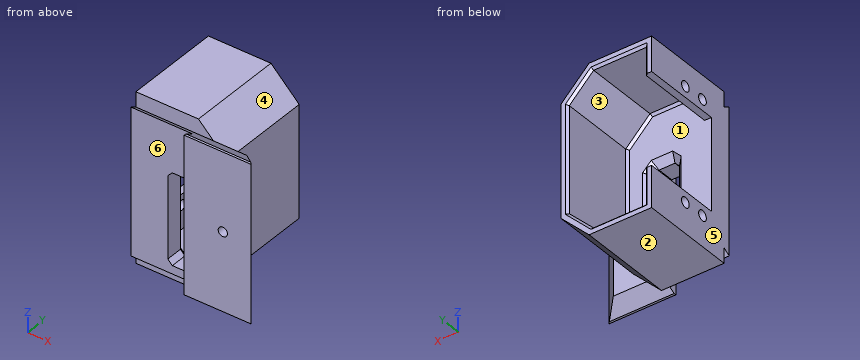
from build123d import *

# Parameters (mm, degrees)
MAIN_FACE_EXTRUDE_DEPTH              = 7.4
MAIN_WALLS_EXTRUDE_DEPTH             = 35
MAIN_WALLS_LOWER_CHAMFER_SIZE        = 1
MAIN_WALLS_ENTRY_CHAMFER_SIZE        = 1
SKETCH4_W                            = 3
SKETCH4_H                            = 40.5
SERVO_MOUNT_CUT_DEPTH                = 35
SERVO_MOUNT_HOLES_REACH              = 72.134
SKETCH5_R                            = 2.25
MOUNT_DOVETAIL_DEPTH                 = 56.8
MOUNT_DOVETAIL_CHAMFER_SIZE          = 8
SKETCH9_W                            = 27.3
SKETCH9_H                            = 68.845299462
DOVETAIL_OFFSET_CUT_DEPTH            = 5
SKETCH10_R                           = 2.05
MOUNT_SCREW_HOLE_DEPTH               = 69.359344643
SKETCH11_R                           = 3.5
MOUNT_SCREW_COUNTERSINK_DEPTH        = 3
MOUNT_SCREW_COUNTERSINK_CHAMFER_SIZE = 1
GEAR_CUT_DEPTH                       = 65.033116432
GEAR_ENTRY_CHAMFER_SIZE              = 3


# Some blends are built 0.0001 mm under size
with BuildPart() as part:
    # Sketch1 → Main Face Extrude (new body)
    with BuildSketch(Plane(origin=(0, 0, 0), x_dir=(1, 0, 0), z_dir=(0, 1, 0))):
        Polygon((-20, 35), (7.542640687, 35), (20, 22.542640687), (20, -26.542640687), (7.542640687, -39), (-20, -39), align=None)
    extrude(amount=MAIN_FACE_EXTRUDE_DEPTH)

    # Sketch3 → Main Walls Extrude (add)
    with BuildSketch(Plane(origin=(0, 7.4, 0), x_dir=(1, 0, 0), z_dir=(0, 1, 0))):
        Polygon((-20, 35), (-20, -39), (7.542640687, -39), (20, -26.542640687), (20, 22.542640687), (7.542640687, 35), align=None)
        Polygon((-17, 32), (-17, -36), (6.3, -36), (17, -25.3), (17, 21.3), (6.3, 32), align=None, mode=Mode.SUBTRACT)
    extrude(amount=MAIN_WALLS_EXTRUDE_DEPTH)

    # Main Walls Lower Chamfer
    main_walls_lower_chamfer_edges = [part.edges().sort_by_distance(p)[0] for p in [
        (-5.35, 7.4, -32),
        (-5.35, 7.4, 36),
        (11.65, 7.4, 30.65),
        (17, 7.4, 2),
        (11.65, 7.4, -26.65),
    ]]
    chamfer(main_walls_lower_chamfer_edges, length=MAIN_WALLS_LOWER_CHAMFER_SIZE)

    # Main Walls Entry Chamfer
    main_walls_entry_chamfer_edges = [part.edges().sort_by_distance(p)[0] for p in [
        (-5.35, 42.4, -32),
        (-17, 42.4, 2),
        (-5.35, 42.4, 36),
        (11.65, 42.4, 30.65),
        (17, 42.4, 2),
        (11.65, 42.4, -26.65),
    ]]
    chamfer(main_walls_entry_chamfer_edges, length=MAIN_WALLS_ENTRY_CHAMFER_SIZE)

    # Sketch4 → Servo Mount Cut (cut)
    with BuildSketch(Plane(origin=(0, 42.4, 0), x_dir=(1, 0, 0), z_dir=(0, 1, 0))):
        with Locations((-18.5, -3.45)):
            Rectangle(SKETCH4_W, SKETCH4_H)
    extrude(amount=-SERVO_MOUNT_CUT_DEPTH, mode=Mode.SUBTRACT)

    # Sketch5 → Servo Mount Holes (cut, up to next)
    with BuildSketch(Plane.ZY.offset(20), mode=Mode.PRIVATE) as servo_mount_holes_sk1:
        with Locations((-21.6, 22.65)):
            Circle(SKETCH5_R)
    servo_mount_holes_tool1 = extrude(servo_mount_holes_sk1.sketch, amount=-SERVO_MOUNT_HOLES_REACH, mode=Mode.PRIVATE) & part.part
    # Sketch5 → Servo Mount Holes (cut, up to next)
    with BuildSketch(Plane.ZY.offset(20), mode=Mode.PRIVATE) as servo_mount_holes_sk2:
        with Locations((-21.6, 12.65)):
            Circle(SKETCH5_R)
    servo_mount_holes_tool2 = extrude(servo_mount_holes_sk2.sketch, amount=-SERVO_MOUNT_HOLES_REACH, mode=Mode.PRIVATE) & part.part
    # Sketch5 → Servo Mount Holes (cut, up to next)
    with BuildSketch(Plane.ZY.offset(20), mode=Mode.PRIVATE) as servo_mount_holes_sk3:
        with Locations((28.5, 22.65)):
            Circle(SKETCH5_R)
    servo_mount_holes_tool3 = extrude(servo_mount_holes_sk3.sketch, amount=-SERVO_MOUNT_HOLES_REACH, mode=Mode.PRIVATE) & part.part
    # Sketch5 → Servo Mount Holes (cut, up to next)
    with BuildSketch(Plane.ZY.offset(20), mode=Mode.PRIVATE) as servo_mount_holes_sk4:
        with Locations((28.5, 12.65)):
            Circle(SKETCH5_R)
    servo_mount_holes_tool4 = extrude(servo_mount_holes_sk4.sketch, amount=-SERVO_MOUNT_HOLES_REACH, mode=Mode.PRIVATE) & part.part
    add(servo_mount_holes_tool1.solids().sort_by_distance((-20, 22.65, -21.6))[0], mode=Mode.SUBTRACT)
    add(servo_mount_holes_tool2.solids().sort_by_distance((-20, 12.65, -21.6))[0], mode=Mode.SUBTRACT)
    add(servo_mount_holes_tool3.solids().sort_by_distance((-20, 22.65, 28.5))[0], mode=Mode.SUBTRACT)
    add(servo_mount_holes_tool4.solids().sort_by_distance((-20, 12.65, 28.5))[0], mode=Mode.SUBTRACT)

    # Sketch8 → Mount Dovetail (add)
    with BuildSketch(Plane.ZY.offset(20)):
        Polygon((-28.381197846, 0), (-32.422649731, -7), (-32.422649731, -8), (36.422649731, -8), (36.422649731, -7), (32.381197846, 0), align=None)
    extrude(amount=-MOUNT_DOVETAIL_DEPTH)

    # Mount Dovetail Chamfer
    mount_dovetail_chamfer_edges = [part.edges().sort_by_distance(p)[0] for p in [
        (36.8, 0, 2),
    ]]
    chamfer(mount_dovetail_chamfer_edges, length=MOUNT_DOVETAIL_CHAMFER_SIZE - 0.0001)  # a hair under: the kernel refuses the full size

    # Sketch9 → Dovetail Offset Cut (cut)
    with BuildSketch(Plane.XZ.offset(8)):
        with Locations((-6.35, 2)):
            Rectangle(SKETCH9_W, SKETCH9_H)
    extrude(amount=-DOVETAIL_OFFSET_CUT_DEPTH, mode=Mode.SUBTRACT)

    # Sketch10 → Mount Screw Hole (cut, through all)
    with BuildSketch(Plane(origin=(0, 0, 0), x_dir=(1, 0, 0), z_dir=(0, 1, 0))):
        with Locations(Location((24.3, -2, 0), (0, 0, 270))):
            Circle(SKETCH10_R)
    extrude(amount=-MOUNT_SCREW_HOLE_DEPTH, mode=Mode.SUBTRACT)

    # Sketch11 → Mount Screw Countersink (cut)
    with BuildSketch(Plane(origin=(0, 0, 0), x_dir=(1, 0, 0), z_dir=(0, 1, 0))):
        with Locations(Location((24.3, -2, 0), (0, 0, 270))):
            Circle(SKETCH11_R)
    extrude(amount=-MOUNT_SCREW_COUNTERSINK_DEPTH, mode=Mode.SUBTRACT)

    # Mount Screw Countersink Chamfer
    # the kernel refuses this chamfer: 1 mm, written as the material it takes off along each edge
    with BuildSketch(Plane(origin=(24.3, 0, 2), x_dir=(0, 0, 1), z_dir=(-1, 0, 0))) as mount_screw_countersink_chamfer_piece_1_section:
        Polygon((3.5 + MOUNT_SCREW_COUNTERSINK_CHAMFER_SIZE, 0), (3.5, -MOUNT_SCREW_COUNTERSINK_CHAMFER_SIZE), (3.5, 0), align=None)
    mount_screw_countersink_chamfer_piece_1 = revolve(axis=Axis((24.3, 0, 2), (0, 1, 0)), mode=Mode.PRIVATE)
    mount_screw_countersink_chamfer_piece_1 = split(mount_screw_countersink_chamfer_piece_1, bisect_by=Plane(origin=(20, -0.483290811, -1.983290811), z_dir=(1, 0, 0)), keep=Keep.TOP, mode=Mode.PRIVATE)
    add(mount_screw_countersink_chamfer_piece_1, mode=Mode.SUBTRACT)

    # Sketch2 → Gear Cut (cut, through all)
    with BuildSketch(Plane(origin=(0, 7.4, 0), x_dir=(1, 0, 0), z_dir=(0, 1, 0))):
        Polygon((-1.7, 26.5), (5.3, 26.5), (7.3, 24.5), (7.3, -11.5), (5.3, -13.5), (-1.7, -13.5), (-3.7, -11.5), (-3.7, 24.5), align=None)
    extrude(amount=-GEAR_CUT_DEPTH, mode=Mode.SUBTRACT)

    # Gear Entry Chamfer
    gear_entry_chamfer_edges = [part.edges().sort_by_distance(p)[0] for p in [
        (-2.7, 7.4, -25.5),
        (-3.7, 7.4, -6.5),
        (-2.7, 7.4, 12.5),
        (1.8, 7.4, 13.5),
        (6.3, 7.4, 12.5),
        (7.3, 7.4, -6.5),
        (6.3, 7.4, -25.5),
        (1.8, 7.4, -26.5),
    ]]
    chamfer(gear_entry_chamfer_edges, length=GEAR_ENTRY_CHAMFER_SIZE)


solid = part.part
Can you work these out from the model? Positions are in its coordinate system, mm. Face numbers are marked on the shaded views. A direction names the side the tool comes from. Give positions to 0.01 mm unless a question says otherwise; leave off trailing zeros. Loops run counter-clockwise (first coordinate to the right, second up) from the corner with the lowest first, then second, coordinate; pieces in that order, holes last. Notation, with made-up numbers: M 67.5,1.25 L 98.5,1.25 A35 cw 98.5,38.25 Z; hole C -14.75,50.5 d6. An arc over 180 degrees is marked long. One line per item, written item: value.
1) Please list where these lines run through material, in increasing order: line 1 (Y direction, x = -19.25, z = 28.5); line 2 (Z direction, x = -12, y = 17); line 3 (X direction, y = 33.5, z = -20).
Geometry check:
line 1: y = -3 to 10.4, 14.9 to 20.4, 24.9 to 42.4
line 2: z = -35 to -32, 36 to 39
line 3: x = -20 to -17, 17 to 20
2) Imagine slicing it at D-D on y = 2. Write out the boundary of the cut face in (x, z), and give its area (3 significant figures).
Geometry check:
outline: M -20,-35 L 7.54,-35 L 20,-22.54 L 20,26.54 L 7.54,39 L -20,39 Z; hole M -3.7,-24.5 L -1.7,-26.5 L 5.3,-26.5 L 7.3,-24.5 L 7.3,11.5 L 5.3,13.5 L -1.7,13.5 L -3.7,11.5 Z
area: 2,370 mm²
3) On a 3-axis mill with a long thin cutter (end or side, diameter ignored), from which of +Z, -Z, +X, -X, +Y, -Y can I reach the whole of each face in a straight line? I mean the marked faces 1 and 2. Say none if no direction works.
Geometry check:
face 1: +Y
face 2: -Z, +X, -X, +Y, -Y
4) Imagine slicing it at B-B on y = 24. Write out the boundary of the cut face in (x, z).
Geometry check:
outline: M -20,-35 L 7.54,-35 L 20,-22.54 L 20,26.54 L 7.54,39 L -20,39 L -20,30.3 L -17,30.3 L -17,36 L 6.3,36 L 17,25.3 L 17,-21.3 L 6.3,-32 L -17,-32 L -17,-23.4 L -20,-23.4 Z; M -20,-19.8 L -17,-19.8 L -17,-16.8 L -20,-16.8 Z; M -20,23.7 L -17,23.7 L -17,26.7 L -20,26.7 Z
5) I'm going to push flat-ended pins straight in: pin 1 (12 mm diameter, centred on x = -13.5, z = -3.5, fed in from +Y); pin 2 (4 mm diameter, centred on y = 17, z = -27.5, fed in from +X); pin 3 (1.5 mm diameter, centred on x = 6, z = 23.5, fed in from -Y). Where does each tip first touch, or does it pass through?
Geometry check:
pin 1: stops at y = 7.4
pin 2: stops at x = 17.04
pin 3: stops at y = -3
6) Imagine slicing it at A-A on z = 2. Count the separate pieces of the cut face and the enclosed holes in it, and give its area (3 significant figures).
Geometry check:
separate pieces: 3
enclosed holes: 0
area: 521 mm²
7) Thinking about a two-plate mould opening in X: for the marked faces 3, 4, 5 and 6, which applies, +X half, -X half, draft (parallel to the pull), parting line (faces both ways), or undercut?
Geometry check:
face 3: undercut
face 4: +X half
face 5: -X half
face 6: draft
8) Imagine slicing it at C-C on x = 24.3. Write out the boundary of the cut face in (y, z).
Geometry check:
outline: M -8,-32.42 L -7,-32.42 L 0,-28.38 L 0,-2.5 L -1,-1.5 L -3,-1.5 L -3,-0.05 L -8,-0.05 Z; M -8,4.05 L -3,4.05 L -3,5.5 L -1,5.5 L 0,6.5 L 0,32.38 L -7,36.42 L -8,36.42 Z
